Print and shaded views of the part. All mm, measured from the part's lowest x, y and z. A direction names the side the tool comes from. Coordinates: 2 decimals unless noted, no trailing zeros. Order: outer loops, then holes, each group sorted by start corner. A loop starts at its lowest first (then second) coordinate and runs counter-clockwise, first axis right, second up. Notation, with made-up numbers: (9, -39.75) -> (67, -39.75) arc R17 ccw to (67, -21.75) -> close; hole circle Ø8 at (-20, 48.25). An arc over 180 degrees is marked (long way). Return JSON: item names as keys, results as strings. Group by question number.
1) Pull direction Y, two halves, no side cores. Call the marked faces 1, 2 and 3: +Y half, -Y half, draft (parallel to the pull), parting line (faces both ways), or undercut.
2) Flat gauge pins, fed straight in: pin 1 (1.8 mm diameter, centred on y = 13, z = 1.5, fed in from -X); pin 2 (0.8 mm diameter, centred on x = 0.5, y = 7.5, fed in from -Z). Where does each tip first touch, or does it go through?
3) Which spindle directions (+Z, -Z, +X, -X, +Y, -Y) get a long thin tool onto all of the face, cutting with end or side? Do the marked faces 4, 5, 6, 7 and 8. Say none if no direction does.
4) Cut at C-C (y = 5). Write the cut outline in (x, z).
5) Cut at A-A (x = 5.5). Write the cut outline in (y, z).
6) Cut at D-D (x = 0.5). Write the cut outline in (y, z).
7) Probe line 1 (Y direction, x = 3.5, z = 5); line 2 (Y direction, x = 5.5, z = 9.1); line 3 (Z direction, x = 4.25, y = 15). List the from-to ranges inside material, lowest first.
8) Cut at B-B (z = 5). Write the cut outline in (x, y), and give its area (3 significant figures).
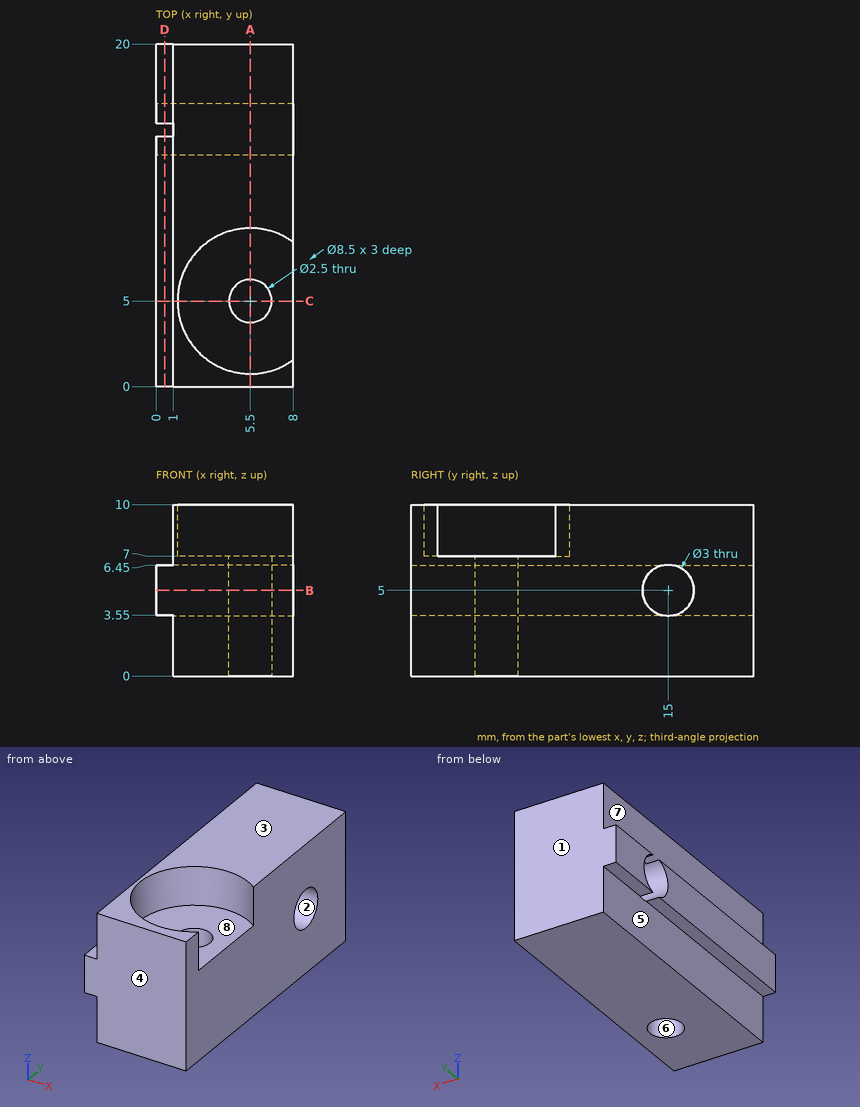
Answers below:
{
 "1": {"face 1": "+Y half", "face 2": "undercut", "face 3": "draft"},
 "2": {"pin 1": "stops at x = 1", "pin 2": "stops at z = 3.55"},
 "3": {"face 4": "+Z, -Z, +X, -X, -Y", "face 5": "-Z, -X, +Y, -Y", "face 6": "+Z, -Z", "face 7": "+Z, -X, +Y, -Y", "face 8": "+Z"},
 "4": {"outline": "(0, 3.55) -> (1, 3.55) -> (1, 0) -> (4.25, 0) -> (4.25, 7) -> (1.25, 7) -> (1.25, 10) -> (1, 10) -> (1, 6.45) -> (0, 6.45) -> close; (6.75, 0) -> (8, 0) -> (8, 7) -> (6.75, 7) -> close"},
 "5": {"outline": "(0, 0) -> (3.75, 0) -> (3.75, 7) -> (0.75, 7) -> (0.75, 10) -> (0, 10) -> close; (6.25, 0) -> (20, 0) -> (20, 10) -> (9.25, 10) -> (9.25, 7) -> (6.25, 7) -> close; hole circle Ø3 at (15, 5)"},
 "6": {"outline": "(0, 3.55) -> (14.62, 3.55) arc R1.5 cw to (14.62, 6.45) -> (0, 6.45) -> close; (15.38, 3.55) -> (20, 3.55) -> (20, 6.45) -> (15.38, 6.45) arc R1.5 cw to start"},
 "7": {"line 1": "y = 0 to 13.5, 16.5 to 20", "line 2": "y = 0 to 0.75, 9.25 to 20", "line 3": "z = 0 to 3.5, 6.5 to 10"},
 "8": {"outline": "(0, 0) -> (8, 0) -> (8, 13.5) -> (0, 13.5) -> close; (0, 16.5) -> (8, 16.5) -> (8, 20) -> (0, 20) -> close; hole circle Ø2.5 at (5.5, 5)", "area": "131 mm^2"}
}
